Could you check a few things on this model? Use its own coordinates, in mm. A direction names the side the tool comes from. Give positions to 0.01 mm unless a question says otherwise; leave off trailing zeros. Loops run counter-clockwise (first coordinate to the right, second up) from the corner with the lowest first, then second, coordinate; pieces in that order, holes last. Notation, with made-up numbers: M 12,-38 L 19,-38 A11 ccw 19,-19 Z; hole C 10.25,3 d5. An arc over 180 degrees is marked long. Return JSON: item names as keys, results as strings. Group by question number.
1. Please list where these lines run through material, in increasing order: line 1 (Z direction, x = 13, y = -19.25); line 2 (X direction, y = -13, z = -29.5); line 3 (Z direction, x = -16, y = -9.25).
2. If we section it at A-A (z = -16): Write out the boundary of the cut face in (x, y).
3. For faces 4 (the flat face through (47.12, -12.52, -4.65)), 5 (the conical face through (10.6, -10.86, -35.75)), 6 (the flat face through (-7.313, -12.522, -22.796)), which set-ups out of +Z, -Z, +X, -X, +Y, -Y let a thin tool reach every point of the face, with its end or its side?
4. If we section it at C-C (y = -3.5): Write out the boundary of the cut face in (x, z), plus the area to 3 significant figures.
5. If we section it at B-B (x = 16): Write out the boundary of the cut face in (y, z), plus the area to 3 significant figures.
6. If we mould it in two halves opening along X, with no side actions, what happens to faces 1 (the flat face through (10, 0, 1)), 2 (the flat face through (18.984, -12.522, 43.375)), 3 (the flat face through (23.11, -12.522, 7.382))? For each: +X half, -X half, draft (parallel to the pull), parting line (faces both ways), or undercut.
7. If we section it at D-D (x = -41.5): Write out the boundary of the cut face in (y, z).
8. For pin 1 (10 mm diameter, centred on y = -19, z = 32, fed in from -X); pin 2 (12 mm diameter, centred on y = -22.5, z = -18, fed in from -X); pin 3 (4 mm diameter, centred on x = -35.5, y = -18.5, fed in from -Z), each with a flat end and sliding along its axis, tell me the tip position at first contact or that it passes through.
```python
from build123d import *

# Parameters (mm, degrees)
F1_DEPTH = 25.4
F3_D     = 2.6
F3_DEPTH = 9.5
F3_TIP   = 0.7811188047


with BuildPart() as f1:
    # F0 (on Front) → F1 (new body)
    with BuildSketch(Plane.XZ):
        with BuildLine():
            ThreePointArc((4.860079591, -11.7332700629), (8.9802561211, -8.9802561211), (11.7332700629, -4.860079591))
            ThreePointArc((11.7332700629, -4.860079591), (12.4559730611, -2.4776470896), (12.7, 0))
            ThreePointArc((12.7, 0), (12.4559730611, 2.4776470896), (11.7332700629, 4.860079591))
            ThreePointArc((11.7332700629, 4.860079591), (8.9802561211, 8.9802561211), (4.860079591, 11.7332700629))
            ThreePointArc((4.860079591, 11.7332700629), (0, 12.7), (-4.860079591, 11.7332700629))
            ThreePointArc((-4.860079591, 11.7332700629), (-8.9802561211, 8.9802561211), (-11.7332700629, 4.860079591))
            ThreePointArc((-11.7332700629, 4.860079591), (-12.7, 0), (-11.7332700629, -4.860079591))
            ThreePointArc((-11.7332700629, -4.860079591), (-8.9802561211, -8.9802561211), (-4.860079591, -11.7332700629))
            ThreePointArc((-4.860079591, -11.7332700629), (0, -12.7), (4.860079591, -11.7332700629))
        make_face()
        with BuildLine():
            ThreePointArc((3.7179078086, 0.83262328), (3.7869069668, 0.4188503605), (3.81, 0))
            ThreePointArc((3.81, 0), (3.7309944269, -0.7718682441), (3.4972542854, -1.5117249959))
            ThreePointArc((3.4972542854, -1.5117249959), (2.8589377627, -2.518446916), (1.9407684924, -3.278645705))
            ThreePointArc((1.9407684924, -3.278645705), (0.83262328, -3.7179078086), (-0.3570249003, -3.7932351918))
            ThreePointArc((-0.3570249003, -3.7932351918), (-1.5117249959, -3.4972542854), (-2.518446916, -2.8589377627))
            ThreePointArc((-2.518446916, -2.8589377627), (-3.278645705, -1.9407684924), (-3.7179078086, -0.83262328))
            ThreePointArc((-3.7179078086, -0.83262328), (-3.7932351918, 0.3570249003), (-3.4972542854, 1.5117249959))
            ThreePointArc((-3.4972542854, 1.5117249959), (-2.8589377627, 2.518446916), (-1.9407684924, 3.278645705))
            ThreePointArc((-1.9407684924, 3.278645705), (-0.83262328, 3.7179078086), (0.3570249003, 3.7932351918))
            ThreePointArc((0.3570249003, 3.7932351918), (1.5117249959, 3.4972542854), (2.518446916, 2.8589377627))
            ThreePointArc((2.518446916, 2.8589377627), (3.278645705, 1.9407684924), (3.7179078086, 0.83262328))
        make_face(mode=Mode.SUBTRACT)
        with BuildLine():
            Line((4.860079591, 11.7332700629), (9.8348340353, 34.1729372384))
            ThreePointArc((9.8348340353, 34.1729372384), (6.6122234033, 34.9398354556), (3.3322324031, 35.4035284571))
            ThreePointArc((3.3322324031, 35.4035284571), (-3.3090097739, 35.4057065219), (-9.8348340353, 34.1729372384))
            Line((-9.8348340353, 34.1729372384), (-4.860079591, 11.7332700629))
            ThreePointArc((-4.860079591, 11.7332700629), (0, 12.7), (4.860079591, 11.7332700629))
        make_face()
        with BuildLine():
            ThreePointArc((34.1729372384, -9.8348340353), (35.2115268641, -4.9660825508), (35.56, 0))
            ThreePointArc((35.56, 0), (35.3444650238, 3.9092700317), (34.7004728807, 7.7711506133))
            ThreePointArc((34.7004728807, 7.7711506133), (34.4521603484, 8.8069431317), (34.1729372384, 9.8348340353))
            Line((34.1729372384, 9.8348340353), (11.7332700629, 4.860079591))
            ThreePointArc((11.7332700629, 4.860079591), (12.4559730611, 2.4776470896), (12.7, 0))
            ThreePointArc((12.7, 0), (12.4559730611, -2.4776470896), (11.7332700629, -4.860079591))
            Line((11.7332700629, -4.860079591), (34.1729372384, -9.8348340353))
        make_face()
        with BuildLine():
            Line((9.8348340353, -34.1729372384), (4.860079591, -11.7332700629))
            ThreePointArc((4.860079591, -11.7332700629), (0, -12.7), (-4.860079591, -11.7332700629))
            Line((-4.860079591, -11.7332700629), (-9.8348340353, -34.1729372384))
            ThreePointArc((-9.8348340353, -34.1729372384), (-6.6122234033, -34.9398354556), (-3.3322324031, -35.4035284571))
            ThreePointArc((-3.3322324031, -35.4035284571), (3.3090097739, -35.4057065219), (9.8348340353, -34.1729372384))
        make_face()
        with BuildLine():
            Line((-34.1729372384, -9.8348340353), (-11.7332700629, -4.860079591))
            ThreePointArc((-11.7332700629, -4.860079591), (-12.7, 0), (-11.7332700629, 4.860079591))
            Line((-11.7332700629, 4.860079591), (-34.1729372384, 9.8348340353))
            ThreePointArc((-34.1729372384, 9.8348340353), (-35.5440477326, 1.0650214928), (-34.7004728807, -7.7711506133))
            ThreePointArc((-34.7004728807, -7.7711506133), (-34.4521603484, -8.8069431317), (-34.1729372384, -9.8348340353))
        make_face()
        with BuildLine():
            Line((-32.6410399972, 14.1094332949), (-45.697455996, 19.7532066129))
            Line((-45.697455996, 19.7532066129), (-48.580662033, -10.8796108586))
            Line((-48.580662033, -10.8796108586), (-34.7004728807, -7.7711506133))
            ThreePointArc((-34.7004728807, -7.7711506133), (-35.5440477326, 1.0650214928), (-34.1729372384, 9.8348340353))
            ThreePointArc((-34.1729372384, 9.8348340353), (-33.475288471, 11.996610429), (-32.6410399972, 14.1094332949))
        make_face()
        with BuildLine():
            Line((-18.1138392628, 30.6006932464), (-25.359374968, 42.840970545))
            Line((-25.359374968, 42.840970545), (-45.697455996, 19.7532066129))
            Line((-45.697455996, 19.7532066129), (-32.6410399972, 14.1094332949))
            ThreePointArc((-32.6410399972, 14.1094332949), (-26.6834191188, 23.5055045495), (-18.1138392628, 30.6006932464))
        make_face()
        with BuildLine():
            Line((3.3322324031, 35.4035284571), (4.6651253644, 49.5649398399))
            Line((4.6651253644, 49.5649398399), (-25.359374968, 42.840970545))
            Line((-25.359374968, 42.840970545), (-18.1138392628, 30.6006932464))
            ThreePointArc((-18.1138392628, 30.6006932464), (-14.0880203211, 32.650287647), (-9.8348340353, 34.1729372384))
            ThreePointArc((-9.8348340353, 34.1729372384), (-3.3090097739, 35.4057065219), (3.3322324031, 35.4035284571))
        make_face()
        with BuildLine():
            ThreePointArc((9.8348340353, 34.1729372384), (17.0856010914, 31.1864687861), (23.5055045495, 26.6834191188))
            Line((23.5055045495, 26.6834191188), (32.9077063694, 37.3567867664))
            Line((32.9077063694, 37.3567867664), (4.6651253644, 49.5649398399))
            Line((4.6651253644, 49.5649398399), (3.3322324031, 35.4035284571))
            ThreePointArc((3.3322324031, 35.4035284571), (6.6122234033, 34.9398354556), (9.8348340353, 34.1729372384))
        make_face()
        with BuildLine():
            ThreePointArc((34.1729372384, 9.8348340353), (34.4521603484, 8.8069431317), (34.7004728807, 7.7711506133))
            Line((34.7004728807, 7.7711506133), (48.580662033, 10.8796108586))
            Line((48.580662033, 10.8796108586), (32.9077063694, 37.3567867664))
            Line((32.9077063694, 37.3567867664), (23.5055045495, 26.6834191188))
            ThreePointArc((23.5055045495, 26.6834191188), (30.0444565036, 19.0222036946), (34.1729372384, 9.8348340353))
        make_face()
        with BuildLine():
            ThreePointArc((34.7004728807, 7.7711506133), (35.3444650238, 3.9092700317), (35.56, 0))
            ThreePointArc((35.56, 0), (35.2115268641, -4.9660825508), (34.1729372384, -9.8348340353))
            ThreePointArc((34.1729372384, -9.8348340353), (33.475288471, -11.996610429), (32.6410399972, -14.1094332949))
            Line((32.6410399972, -14.1094332949), (45.697455996, -19.7532066129))
            Line((45.697455996, -19.7532066129), (48.580662033, 10.8796108586))
            Line((48.580662033, 10.8796108586), (34.7004728807, 7.7711506133))
        make_face()
        with BuildLine():
            Line((45.697455996, -19.7532066129), (32.6410399972, -14.1094332949))
            ThreePointArc((32.6410399972, -14.1094332949), (26.6834191188, -23.5055045495), (18.1138392628, -30.6006932464))
            Line((18.1138392628, -30.6006932464), (25.359374968, -42.840970545))
            Line((25.359374968, -42.840970545), (45.697455996, -19.7532066129))
        make_face()
        with BuildLine():
            Line((25.359374968, -42.840970545), (18.1138392628, -30.6006932464))
            ThreePointArc((18.1138392628, -30.6006932464), (14.0880203211, -32.650287647), (9.8348340353, -34.1729372384))
            ThreePointArc((9.8348340353, -34.1729372384), (3.3090097739, -35.4057065219), (-3.3322324031, -35.4035284571))
            Line((-3.3322324031, -35.4035284571), (-4.6651253644, -49.5649398399))
            Line((-4.6651253644, -49.5649398399), (25.359374968, -42.840970545))
        make_face()
        with BuildLine():
            Line((-32.9077063694, -37.3567867664), (-4.6651253644, -49.5649398399))
            Line((-4.6651253644, -49.5649398399), (-3.3322324031, -35.4035284571))
            ThreePointArc((-3.3322324031, -35.4035284571), (-6.6122234033, -34.9398354556), (-9.8348340353, -34.1729372384))
            ThreePointArc((-9.8348340353, -34.1729372384), (-17.0856010914, -31.1864687861), (-23.5055045495, -26.6834191188))
            Line((-23.5055045495, -26.6834191188), (-32.9077063694, -37.3567867664))
        make_face()
        with BuildLine():
            Line((-48.580662033, -10.8796108586), (-32.9077063694, -37.3567867664))
            Line((-32.9077063694, -37.3567867664), (-23.5055045495, -26.6834191188))
            ThreePointArc((-23.5055045495, -26.6834191188), (-30.0444565036, -19.0222036946), (-34.1729372384, -9.8348340353))
            ThreePointArc((-34.1729372384, -9.8348340353), (-34.4521603484, -8.8069431317), (-34.7004728807, -7.7711506133))
            Line((-34.7004728807, -7.7711506133), (-48.580662033, -10.8796108586))
        make_face()
    extrude(amount=F1_DEPTH)

    # F3
    with Locations(Plane(origin=(10.3471248018, 0, -46.2029551924), x_dir=(0.9758288212, 0, 0.218536294), z_dir=(0.218536294, 0, -0.9758288212))):
        with Locations((-2.3135205983, 14.6098749805), (2.3135205983, 14.6098749805), (2.3135205983, 10.7901250195), (-2.3135205983, 10.7901250195)):
            Hole(F3_D / 2, depth=F3_DEPTH)
            with Locations((0, 0, -(F3_DEPTH + F3_TIP / 2))):  # 118° drill point
                Cone(0, F3_D / 2, F3_TIP, mode=Mode.SUBTRACT)


solid = f1.part
```
Answer:
{
 "1": {"line 1": "z = -45.61 to -33.1, -5.14 to 5.14, 33.1 to 45.96", "line 2": "x = -37.56 to -19.86, -8.8 to 8.8, 19.86 to 37.11", "line 3": "z = -44.67 to -31.76, -5.81 to 5.81, 31.76 to 44.94"},
 "2": {"outline": "M -45.55,-25.4 L -31.76,-25.4 L -31.76,0 L -45.55,0 Z; M -5.81,-25.4 L 5.81,-25.4 L 5.81,0 L -5.81,0 Z; M 31.76,-25.4 L 46.05,-25.4 L 46.05,0 L 31.76,0 Z"},
 "3": {"face 4": "-Z, +X, +Y, -Y", "face 5": "none", "face 6": "+Y, -Y"},
 "4": {"outline": "M -48.58,-10.88 L -32.91,-37.36 L -4.67,-49.56 L 25.36,-42.84 L 45.7,-19.75 L 48.58,10.88 L 32.91,37.36 L 4.67,49.56 L -25.36,42.84 L -45.7,19.75 Z; hole M -34.17,-9.83 A35.56 ccw -9.83,-34.17 L -4.86,-11.73 A12.7 cw -11.73,-4.86 Z; hole M -34.17,9.83 L -11.73,4.86 A12.7 cw -4.86,11.73 L -9.83,34.17 A35.56 ccw Z; hole C 0,0 d7.62; hole M 4.86,-11.73 L 9.83,-34.17 A35.56 ccw 34.17,-9.83 L 11.73,-4.86 A12.7 cw Z; hole M 4.86,11.73 A12.7 cw 11.73,4.86 L 34.17,9.83 A35.56 ccw 9.83,34.17 Z", "area": "5,140 mm²"},
 "5": {"outline": "M -25.4,-44.94 L 0,-44.94 L 0,-31.76 L -25.4,-31.76 Z; M -25.4,-5.81 L 0,-5.81 L 0,5.81 L -25.4,5.81 Z; M -25.4,31.76 L 0,31.76 L 0,44.67 L -25.4,44.67 Z", "area": "958 mm²"},
 "6": {"face 1": "draft", "face 2": "+X half", "face 3": "undercut"},
 "7": {"outline": "M -25.4,-22.84 L 0,-22.84 L 0,24.52 L -25.4,24.52 Z"},
 "8": {"pin 1": "stops at x = -39.31", "pin 2": "stops at x = -47.92", "pin 3": "stops at z = -36.36"}
}
